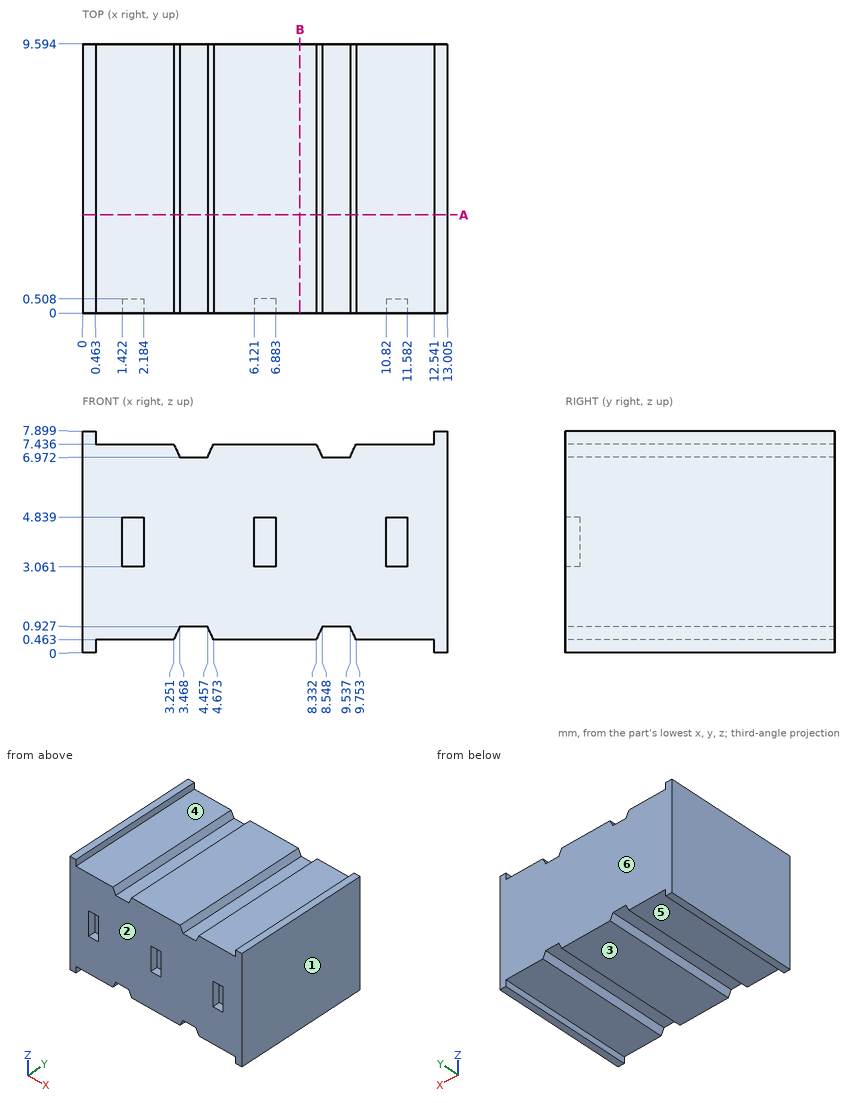
For this review, use the dimensioned drawing (mm, ordinates from the lowest corner) and the shaded views. A direction names the side the tool comes from. Round coordinates to 2 decimals unless told otherwise and drop trailing zeros. Write each loop counter-clockwise with the first axis right and the second up, starting at its lowest first coordinate (ties: lowest second). Pieces come first, ordered by that corner, then holes. Notation, with made-up numbers: M 51,-11.75 L 79,-11.75 A18 ccw 79,4.25 Z; hole C -40,67 d5. An arc over 180 degrees is marked long. Write item = value, one per line. Start each with the question number.
(1) For line 1 along X through (y, z) = (4.25, 7.25) (1 decimal); line 2 along X through (y, z) = (6.25, 7.75) (1 decimal); line 3 along Z through (x, y) = (5, 7.25) (1 decimal), list the stretches that pass through material, from the lowest coordinate up.
(2) For the marked faces 4, 5 and 6, list the 3-axis set-ups (+Z, -Z, +X, -X, +Y, -Y) from which the entire face can be reached by the end or side of a thin tool; tool diameter is ignored.
(3) The part is to be moulded in two halves that separate along X. For the marked faces 1, 2 and 3, say which applies: +X half, -X half, draft (parallel to the pull), parting line (faces both ways), or undercut.
(4) We need section B-B (x = 7.75). Give the boundary of the cut face in (y, z) (1 decimal).
(5) We need section A-A (y = 3.5). Give the boundary of the cut face in (x, z) (1 decimal).
(6) Clearance check with flat-ended pins moving along their axes: pin 1 Ø1 at (y, z) = (1, 6) entering from -X; pin 2 Ø0.5 at (x, y) = (9, 3.5) entering from -Z; pin 3 Ø1.4 at (x, y) = (2, 4) entering from +Z; pin 4 Ø1.1 at (x, y) = (4, 4.5) entering from +Z (1 decimal). State where each tip first meets the part, or that it passes through.
Results found:
q1.line_1 = 0 to 3.3, 4.6 to 8.4, 9.7 to 13
q1.line_2 = 0 to 0.5, 12.5 to 13
q1.line_3 = 0.5 to 7.4
q2.face_4 = +Z, +Y, -Y
q2.face_5 = -Z, +Y, -Y
q2.face_6 = +Z, -Z, +X, -X, +Y
q3.face_1 = +X half
q3.face_2 = draft
q3.face_3 = undercut
q4.outline = M 0,0.5 L 9.6,0.5 L 9.6,7.4 L 0,7.4 Z
q5.outline = M 0,0 L 0.5,0 L 0.5,0.5 L 3.3,0.5 L 3.5,0.9 L 4.5,0.9 L 4.7,0.5 L 8.3,0.5 L 8.5,0.9 L 9.5,0.9 L 9.8,0.5 L 12.5,0.5 L 12.5,0 L 13,0 L 13,7.9 L 12.5,7.9 L 12.5,7.4 L 9.8,7.4 L 9.5,7 L 8.5,7 L 8.3,7.4 L 4.7,7.4 L 4.5,7 L 3.5,7 L 3.3,7.4 L 0.5,7.4 L 0.5,7.9 L 0,7.9 Z
q6.pin_1 = 0
q6.pin_2 = 0.93
q6.pin_3 = 7.44
q6.pin_4 = 7.2
